Here's how the part is built. I have some questions about the finished solid (model axes, mm). Coordinates: 2 decimals unless noted, no trailing zeros. Use CSV: the item, a comma, the result in double quotes. Start each with the question number.
from build123d import *

# Parameters (mm, degrees)
ESQUISSE3_W                       = 44
ESQUISSE3_H                       = 6
ENL_V_MAT_EXTRU_3_DEPTH           = 15
ENL_V_MAT_EXTRU_3_DRAFT           = 1
ENL_V_MAT_EXTRU_3_PROFILE_2_DEPTH = 15
ENL_V_MAT_EXTRU_3_PROFILE_2_DRAFT = 1
ENL_V_MAT_EXTRU_3_PROFILE_3_DEPTH = 15
ENL_V_MAT_EXTRU_3_PROFILE_3_DRAFT = 1
ENL_V_MAT_EXTRU_3_PROFILE_4_DEPTH = 15
ENL_V_MAT_EXTRU_3_PROFILE_4_DRAFT = 1
CONG_1_R                          = 3


with BuildPart() as part:
    # Esquisse1 → Lissage1 section 0
    with BuildSketch(Plane.XY):
        with BuildLine():
            Line((-27.75, 27.75), (27.75, 27.75))
            Line((27.75, 27.75), (27.75, -27.75))
            Line((27.75, -27.75), (-27.75, -27.75))
            Line((-27.75, -27.75), (-27.75, 27.75))
        make_face()
    # Esquisse2 → Lissage1 section 1
    with BuildSketch(Plane.XY.offset(-20)):
        with BuildLine():
            Line((-30.33229437, 30.25), (30.16770563, 30.249999987))
            Line((30.16770563, 30.249999987), (30.166474554, -30.25))
            Line((30.166474554, -30.25), (-30.333525446, -30.25))
            Line((-30.333525446, -30.25), (-30.33229437, 30.25))
        make_face()
    loft()


with BuildPart() as enl_v_mat_extru_3_tool:
    # Esquisse3 → Enlèv. mat.-Extru.3 (with draft: the straight prism first)
    with BuildSketch(Plane.XY.offset(-20)):
        with Locations((0, -6.65)):
            Rectangle(ESQUISSE3_W, ESQUISSE3_H)
    extrude(amount=ENL_V_MAT_EXTRU_3_DEPTH)
    # Enlèv. mat.-Extru.3: the draft: its side faces are tilted about the plane it starts from
    enl_v_mat_extru_3_sides = [enl_v_mat_extru_3_tool.faces().sort_by_distance(p)[0] for p in [
        (0, -9.65, -12.5),
        (22, -6.65, -12.5),
        (0, -3.65, -12.5),
        (-22, -6.65, -12.5),
    ]]
    draft(enl_v_mat_extru_3_sides, Plane.XY.offset(-20), ENL_V_MAT_EXTRU_3_DRAFT)


with BuildPart() as part_1:
    add(part.part)

    # Enlèv. mat.-Extru.3: cut by enl_v_mat_extru_3_tool
    add(enl_v_mat_extru_3_tool.part, mode=Mode.SUBTRACT)


with BuildPart() as enl_v_mat_extru_3_profile_2_tool:
    # Esquisse3 → Enlèv. mat.-Extru.3 profile 2 (with draft: the straight prism first)
    with BuildSketch(Plane.XY.offset(-20)):
        with Locations((0, -19.95)):
            Rectangle(ESQUISSE3_W, ESQUISSE3_H)
    extrude(amount=ENL_V_MAT_EXTRU_3_PROFILE_2_DEPTH)
    # Enlèv. mat.-Extru.3 profile 2: the draft: its side faces are tilted about the plane it starts from
    enl_v_mat_extru_3_profile_2_sides = [enl_v_mat_extru_3_profile_2_tool.faces().sort_by_distance(p)[0] for p in [
        (0, -22.95, -12.5),
        (22, -19.95, -12.5),
        (0, -16.95, -12.5),
        (-22, -19.95, -12.5),
    ]]
    draft(enl_v_mat_extru_3_profile_2_sides, Plane.XY.offset(-20), ENL_V_MAT_EXTRU_3_PROFILE_2_DRAFT)


with BuildPart() as part_2:
    add(part_1.part)

    # Enlèv. mat.-Extru.3 profile 2: cut by enl_v_mat_extru_3_profile_2_tool
    add(enl_v_mat_extru_3_profile_2_tool.part, mode=Mode.SUBTRACT)


with BuildPart() as enl_v_mat_extru_3_profile_3_tool:
    # Esquisse3 → Enlèv. mat.-Extru.3 profile 3 (with draft: the straight prism first)
    with BuildSketch(Plane.XY.offset(-20)):
        with Locations((0, 6.65)):
            Rectangle(ESQUISSE3_W, ESQUISSE3_H)
    extrude(amount=ENL_V_MAT_EXTRU_3_PROFILE_3_DEPTH)
    # Enlèv. mat.-Extru.3 profile 3: the draft: its side faces are tilted about the plane it starts from
    enl_v_mat_extru_3_profile_3_sides = [enl_v_mat_extru_3_profile_3_tool.faces().sort_by_distance(p)[0] for p in [
        (0, 3.65, -12.5),
        (22, 6.65, -12.5),
        (0, 9.65, -12.5),
        (-22, 6.65, -12.5),
    ]]
    draft(enl_v_mat_extru_3_profile_3_sides, Plane.XY.offset(-20), ENL_V_MAT_EXTRU_3_PROFILE_3_DRAFT)


with BuildPart() as part_3:
    add(part_2.part)

    # Enlèv. mat.-Extru.3 profile 3: cut by enl_v_mat_extru_3_profile_3_tool
    add(enl_v_mat_extru_3_profile_3_tool.part, mode=Mode.SUBTRACT)


with BuildPart() as enl_v_mat_extru_3_profile_4_tool:
    # Esquisse3 → Enlèv. mat.-Extru.3 profile 4 (with draft: the straight prism first)
    with BuildSketch(Plane.XY.offset(-20)):
        with Locations((0, 19.95)):
            Rectangle(ESQUISSE3_W, ESQUISSE3_H)
    extrude(amount=ENL_V_MAT_EXTRU_3_PROFILE_4_DEPTH)
    # Enlèv. mat.-Extru.3 profile 4: the draft: its side faces are tilted about the plane it starts from
    enl_v_mat_extru_3_profile_4_sides = [enl_v_mat_extru_3_profile_4_tool.faces().sort_by_distance(p)[0] for p in [
        (0, 16.95, -12.5),
        (22, 19.95, -12.5),
        (0, 22.95, -12.5),
        (-22, 19.95, -12.5),
    ]]
    draft(enl_v_mat_extru_3_profile_4_sides, Plane.XY.offset(-20), ENL_V_MAT_EXTRU_3_PROFILE_4_DRAFT)


with BuildPart() as part_4:
    add(part_3.part)

    # Enlèv. mat.-Extru.3 profile 4: cut by enl_v_mat_extru_3_profile_4_tool
    add(enl_v_mat_extru_3_profile_4_tool.part, mode=Mode.SUBTRACT)

    # Congé1
    cong_1_edges = [part_4.edges().sort_by_distance(p)[0] for p in [
        (-29.041147185, 29, -10),
        (-29.041762723, -29, -10),
        (28.958852815, 28.999999994, -10),
        (28.958237277, -29, -10),
    ]]
    fillet(cong_1_edges, radius=CONG_1_R)


solid = part_4.part
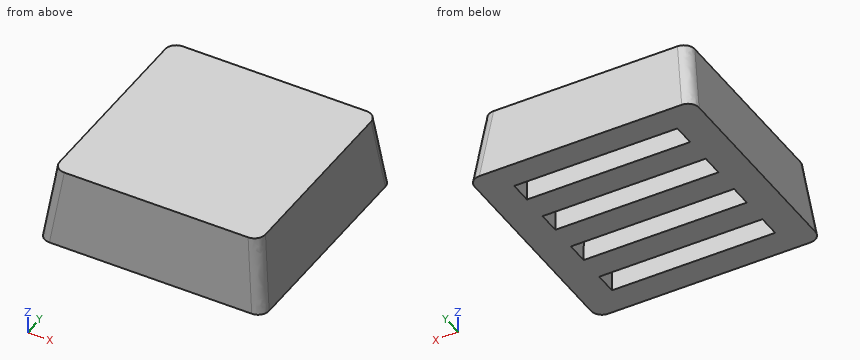
1) For P1, Ø1.5, axis at x = 15.5, y = 10.5, coming from the +Z side; P2, Ø1.6, axis at x = -3, y = 6.5, coming from the -Z side; P3, Ø3, axis at x = -22.5, z = -3.5, coming from the +Y side (3 decimals); P4, Ø8, axis at x = -10.5, z = -2, coming from the +Y side, each with a flat end and sliding along its axis, tell me the tip position at first contact or that it passes through.
2) I want a section at A-A, the plane z = -9. State how many separate pieces and enclosed holes the cut face has, plus the area to 3 significant figures.
3) Please list where these lines run through material, in increasing order: L1, parallel to Y at x = 0, z = -14.5; L2, parallel to Z at x = 11, y = -5.5; L3, parallel to Y at x = 13, z = -6. Write a range as [from, to].
Return value:
1,P1,"stops at z = 0"
1,P2,"stops at z = -5"
1,P3,"stops at y = 28.375"
1,P4,"stops at y = 28.5"
2,separate pieces,"1"
2,enclosed holes,"4"
2,area,"2,350 mm²"
3,L1,"y = [-29.56, -22.85], [-17.05, -9.55], [-3.75, 3.75], [9.55, 17.05], [22.85, 29.56]"
3,L2,"z = [-5, 0]"
3,L3,"y = [-28.5, -22.71], [-17.19, -9.41], [-3.89, 3.89], [9.41, 17.19], [22.71, 28.5]"
